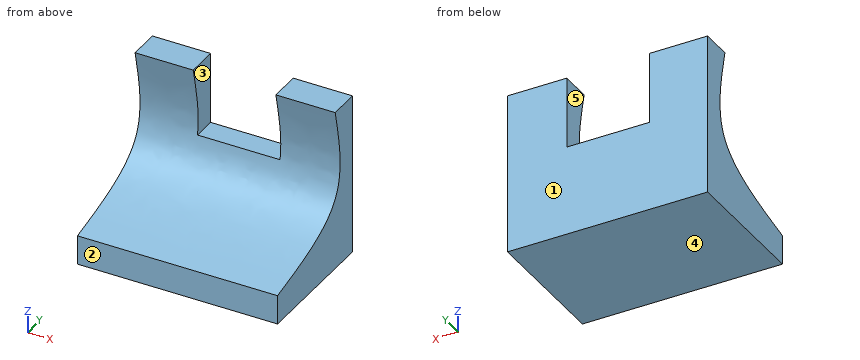
from build123d import *

# Parameters (mm, degrees)
F0_W     = 75.6122842431
F0_H     = 61.000533402
F1_DEPTH = 50.8
F3_DEPTH = 76.2
F4_W     = 31.2095750123
F4_H     = 26.9537232816
F5_DEPTH = 25.4


with BuildPart() as f1:
    # F0 (on Front) → F1 (new body)
    with BuildSketch(Plane.XZ):
        with Locations((37.8061421216, 30.500266701)):
            Rectangle(F0_W, F0_H)
    extrude(amount=F1_DEPTH)

    # F2 (on face) → F3 (cut)
    with BuildSketch(Plane(origin=(0, 0, 0), x_dir=(0, -1, 0), z_dir=(-1, 0, 0))):
        with BuildLine():
            Line((50.8, 61.000533402), (11.7745203897, 61.000533402))
            add(Edge.make_bspline(
                [(11.7745203897, 61.000533402), (8.9290710165, 48.3611461348), (2.8734064272, 21.462094399), (34.1955670512, 14.6672699688), (50.8, 11.0652130097)],
                knots=[0, 0, 0, 0, 0.4698822617, 1, 1, 1, 1], degree=3))
            Line((50.8, 11.0652130097), (50.8, 61.000533402))
        make_face()
    extrude(amount=-F3_DEPTH, mode=Mode.SUBTRACT)

    # F4 (on face) → F5 (cut)
    with BuildSketch(Plane(origin=(0, 0, 0), x_dir=(-1, 0, 0), z_dir=(0, 1, 0))):
        with Locations((-37.5933526084, 47.5236717612)):
            Rectangle(F4_W, F4_H)
    extrude(amount=-F5_DEPTH, mode=Mode.SUBTRACT)


solid = f1.part
Build history of the part. All positions in model axes, mm. Face numbers are marked on the shaded views. A direction names the side the tool comes from. Give positions to 0.01 mm unless a question says otherwise; leave off trailing zeros. Loops run counter-clockwise (first coordinate to the right, second up) from the corner with the lowest first, then second, coordinate; pieces in that order, holes last. Notation, with made-up numbers: (88.5, 84.5) - (124.5, 84.5) arc R22 cw to (124.5, 107.5) - close; hole circle Ø6 at (17, -6). An arc over 180 degrees is marked (long way). Write item = value, one per line. Start each with the question number.
1) Tool access for the marked faces 4 and 5: list every direction of +Z, -Z, +X, -X, +Y, -Y with a clear straight run to the whole face (end or side of a thin tool).
2) Pull direction Y, two halves, no side cores. Call the marked faces 1, 2 and 3: +Y half, -Y half, draft (parallel to the pull), parting line (faces both ways), or undercut.
3) Probe probe 1 along Z at (x, y) = (25.5, -39.5); probe 2 along Z at (x, y) = (17.5, -33.5); probe 3 along Y at (x, z) = (12, 25). List the from-to ranges inside material, lowest first. Write a range as from..to.
4) Drop flat-ended pins along their axis: pin 1 Ø1.5 at (x, z) = (10, 41.5) entering from -Y; pin 2 Ø4 at (x, z) = (54, 35) entering from -Y; pin 3 Ø7 at (x, y) = (30.5, -3.5) entering from +Z. Give the stop position or say it passes through.
5) Band-saw the part on A-A on y = -5. Give the cut face in (x, z), plus the area to 3 significant figures.
Final values:
q1.face_4 = -Z, +X, -X, +Y, -Y
q1.face_5 = +Z, +Y, -Y
q2.face_1 = +Y half
q2.face_2 = -Y half
q2.face_3 = draft
q3.probe_1 = 0..13.61
q3.probe_2 = 0..15.18
q3.probe_3 = -13.54..0
q4.pin_1 = -8.52
q4.pin_2 = -9.16
q4.pin_3 = 34.05
q5.outline = (0, 0) - (75.61, 0) - (75.61, 61) - (53.2, 61) - (53.2, 34.05) - (21.99, 34.05) - (21.99, 61) - (0, 61) - close
q5.area = 3,770 mm²
